from build123d import *

# Parameters (mm, degrees)
SKETCH1_W          = 195
SKETCH1_H          = 45
SHAPE_DEPTH        = 1300
CUT_EXTRUDE1_REACH = 47
SKETCH2_R          = 12.5


with BuildPart() as part:
    # Sketch1 → Shape (new body)
    with BuildSketch(Plane(origin=(0, 0, 0), x_dir=(1, 0, 0), z_dir=(0, 1, 0))):
        Rectangle(SKETCH1_W, SKETCH1_H)
    extrude(amount=SHAPE_DEPTH)

    # Sketch2 → Cut-Extrude1 (cut, up to next)
    with BuildSketch(Plane.XY.offset(22.5), mode=Mode.PRIVATE) as cut_extrude1_sk1:
        with Locations((0, 180)):
            Circle(SKETCH2_R)
    cut_extrude1_tool1 = extrude(cut_extrude1_sk1.sketch, amount=-CUT_EXTRUDE1_REACH, mode=Mode.PRIVATE) & part.part
    add(cut_extrude1_tool1.solids().sort_by_distance((0, 180, 22.5))[0], mode=Mode.SUBTRACT)


solid = part.part
For this review, take the finished solid that the model builds, in its own axes (mm). Round coordinates to 2 decimals unless told otherwise and drop trailing zeros. Write each loop counter-clockwise with the first axis right and the second up, starting at its lowest first coordinate (ties: lowest second). Pieces come first, ordered by that corner, then holes. Notation, with made-up numbers: (66.25, 49.25) - (107.25, 49.25) arc R8 cw to (107.25, 58.25) - close; hole circle Ø11 at (73, 89.5). An arc over 180 degrees is marked (long way). Write item = value, one per line. Start each with the question number.
1. For pin 1 Ø20 at (x, y) = (0, 180) entering from +Z, flat-tipped, find the tip position at first contact; note if it passes through.
2. Consider section A-A on y = 180. State the section outline as (x, z) points.
3. Consider section B-B on x = 0. State the section outline as (y, z) points.
4. Wall thickness on L1, parallel to Y at x = 0, z = -6; L2, parallel to Y at x = 5.5, z = 4: over which ranges is each line inside the solid? List them lowest first.
5. Draft analysis for pull direction Y (two halves, no side actions). For faces 1 (the face through (-1.627, 192.394, 0.315)), 2 (the face through (-1, 641, 22.5)), 3 (the face through (-1, 0, 0)), state which applies: released by +Y, released by -Y, zero draft, split by the parting line, or undercut.
Evaluation:
q1.pin_1 = through
q2.outline = (-97.5, -22.5) - (-12.5, -22.5) - (-12.5, 22.5) - (-97.5, 22.5) - close; (12.5, -22.5) - (97.5, -22.5) - (97.5, 22.5) - (12.5, 22.5) - close
q3.outline = (0, -22.5) - (167.5, -22.5) - (167.5, 22.5) - (0, 22.5) - close; (192.5, -22.5) - (1300, -22.5) - (1300, 22.5) - (192.5, 22.5) - close
q4.L1 = 0 to 167.5, 192.5 to 1300
q4.L2 = 0 to 168.78, 191.22 to 1300
q5.face_1 = undercut
q5.face_2 = zero draft
q5.face_3 = released by -Y
